Input: dimensioned drawing with shaded views. Units: mm. Origin: part minimum x, y, z. Give positions to 0.01 mm unless a question says otherwise; leave off trailing zeros. Order: outer loops, then holes, each group sorted by start corner. A loop starts at its lowest first (then second) coordinate and runs counter-clockwise, first axis right, second up. Notation, with made-up numbers: (15, -9.75) -> (74, -9.75) arc R20 cw to (74, 23.25) -> close; hole circle Ø11 at (85, 38.5). An arc over 180 degrees is marked (long way). Use CSV: the item, a comma, the result in double quotes.
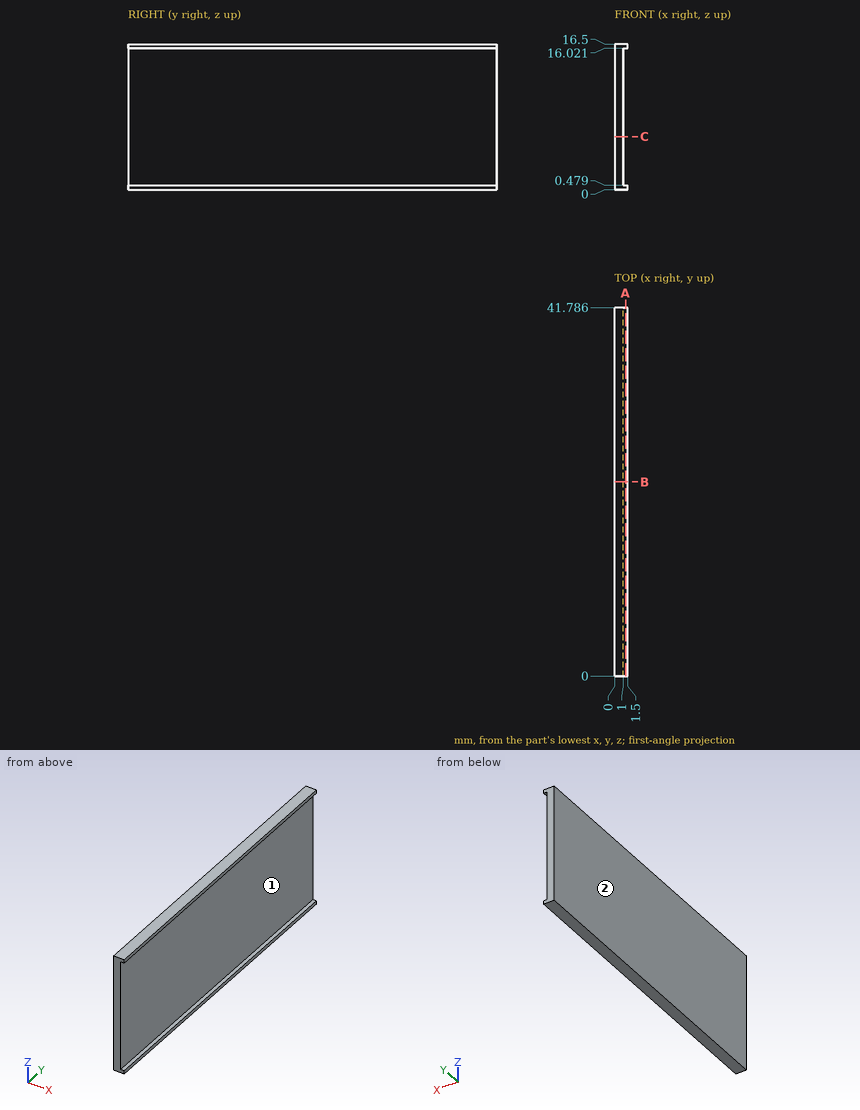
1. Section query A-A on x = 1.25. Return loops of the section in (y, z).
Answer below:
outline,"(0, 0) -> (41.79, 0) -> (41.79, 0.48) -> (0, 0.48) -> close; (0, 16.02) -> (41.79, 16.02) -> (41.79, 16.5) -> (0, 16.5) -> close"
2. Pin query (flat end, axial travel): P1, Ø8, axis at y = 29.5, z = 10, coming from the +X side. Return the tip coordinate at first contact, or that it passes through.
Answer below:
P1,"stops at x = 1"
3. Section query B-B on y = 22. Return loops of the section in (x, z).
Answer below:
outline,"(0, 0) -> (1.5, 0) -> (1.5, 0.48) -> (1, 0.48) -> (1, 16.02) -> (1.5, 16.02) -> (1.5, 16.5) -> (0, 16.5) -> close"
4. Mould query, pull axis Z, two halves, no side actions, for the marked faces 1 and 2. Classes: released by +Z, released by -Z, zero draft, split by the parting line, or undercut.
Answer below:
face 1,"undercut"
face 2,"zero draft"
5. Section query C-C on z = 6. Return loops of the section in (x, y).
Answer below:
outline,"(0, 0) -> (1, 0) -> (1, 41.79) -> (0, 41.79) -> close"
6. Ray query, line 1 along X through (y, z) = (35.5, 4.5); line 2 along Z through (x, y) = (1.15, 34.5). Return the intervals inside material, ascending.
Answer below:
line 1,"x = 0 to 1"
line 2,"z = 0 to 0.48, 16.02 to 16.5"
